CAD build for the part. Positions are in the model's coordinates, mm. Face numbers are marked on the shaded views. A direction names the side the tool comes from. Round coordinates to 2 decimals unless told otherwise and drop trailing zeros. Order: outer loops, then holes, each group sorted by start corner. A loop starts at its lowest first (then second) coordinate and runs counter-clockwise, first axis right, second up. Notation, with made-up numbers: M 87,40.25 L 99,40.25 A26 ccw 99,70.25 Z; hole C 35,-19 d11. An arc over 180 degrees is marked long. Put each result on its own line as item: value.
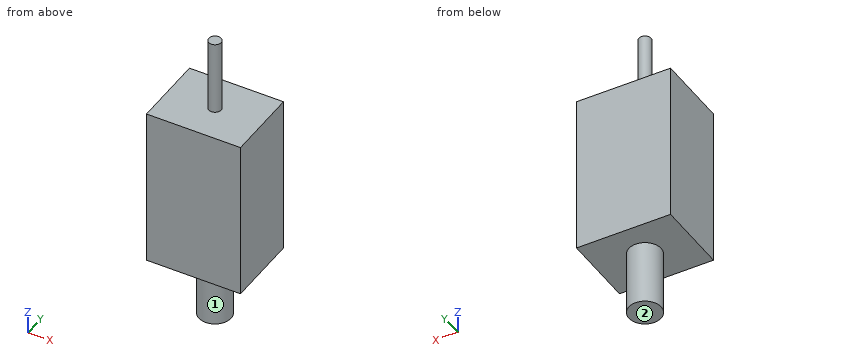
```python
from build123d import *

# Parameters (mm, degrees)
SKETCH1_W           = 38
SKETCH1_H           = 30
BOSS_EXTRUDE1_DEPTH = 65
SKETCH2_R           = 2.5
BOSS_EXTRUDE2_DEPTH = 30
SKETCH3_R           = 6.5
BOSS_EXTRUDE3_DEPTH = 26


with BuildPart() as part:
    # Sketch1 → Boss-Extrude1 (new body)
    with BuildSketch(Plane.XY):
        Rectangle(SKETCH1_W, SKETCH1_H)
    extrude(amount=BOSS_EXTRUDE1_DEPTH)

    # Sketch2 → Boss-Extrude2 (add)
    with BuildSketch(Plane.XY.offset(65)):
        with Locations(Location((0, 0, 0), (0, 0, 180))):
            Circle(SKETCH2_R)
    extrude(amount=BOSS_EXTRUDE2_DEPTH)

    # Sketch3 → Boss-Extrude3 (add)
    with BuildSketch(Plane(origin=(0, 0, 0), x_dir=(-1, 0, 0), z_dir=(0, 0, -1))):
        with Locations(Location((0, 0, 0), (0, 0, 180))):
            Circle(SKETCH3_R)
    extrude(amount=BOSS_EXTRUDE3_DEPTH)


solid = part.part
```
Item 1: Band-saw the part on A-A on y = 0. Give the cut face in (x, z).
Answers below:
outline: M -19,0 L -6.5,0 L -6.5,-26 L 6.5,-26 L 6.5,0 L 19,0 L 19,65 L 2.5,65 L 2.5,95 L -2.5,95 L -2.5,65 L -19,65 Z
Item 2: Band-saw the part on B-B on x = 0. Give the cut face in (y, z).
Answers below:
outline: M -15,0 L -6.5,0 L -6.5,-26 L 6.5,-26 L 6.5,0 L 15,0 L 15,65 L 2.5,65 L 2.5,95 L -2.5,95 L -2.5,65 L -15,65 Z
Item 3: Pin check, flat tips, straight feed: P1, Ø6, axis at x = -13, y = -4.5, coming from the -Z side; P2, Ø10, axis at x = -5.5, y = -10, coming from the +Z side. Stop position of each tip, or through.
Answers below:
P1: z = 0
P2: z = 65
Item 4: Probe line 1 along Z through (x, y) = (-6, -11.75); line 2 along Z through (x, y) = (3, 3.5); line 3 along X through (y, z) = (0.75, 89). List the from-to ranges inside material, lowest first. Write a range as [from, to].
Answers below:
line 1: [0, 65]
line 2: [-26, 65]
line 3: [-2.38, 2.38]
Item 5: Band-saw the part on C-C on y = -10.5. Give the cut face in (x, z).
Answers below:
outline: M -19,0 L 19,0 L 19,65 L -19,65 Z
Item 6: Tool access for the marked faces 1 and 2: list every direction of +Z, -Z, +X, -X, +Y, -Y with a clear straight run to the whole face (end or side of a thin tool).
Answers below:
face 1: -Z
face 2: -Z, +X, -X, +Y, -Y
